Here's how the part is built. I have some questions about the finished solid (model axes, mm). A direction names the side the tool comes from. Coordinates: 2 decimals unless noted, no trailing zeros. Write each loop counter-clockwise with the first axis right and the second up, starting at its lowest first coordinate (ties: lowest second). Pieces come first, ordered by that corner, then holes. Notation, with made-up numbers: (76.25, 9) -> (129.25, 9) arc R16 ccw to (129.25, 29) -> close; hole circle Ø6 at (54, 84.25). An arc over 180 degrees is marked (long way). Use a Markdown table: item, result. Add a question column.
Item 1: If I drill on line 1 along Y through (x, z) = (0, 33.5); line 2 along Z through (x, y) = (-28.5, 17); line 3 along Y through (x, z) = (5, 60), over which ranges is the centre line in solid material (lowest first)? Write a range as from..to.
Item 2: If we mould it in two halves opening along X, with no side actions, what happens to faces 3 (the flat face through (-12, -4, 160)), 4 (the conical face through (34.327, -7.623, 0.243)), 5 (the cylindrical face through (-12.19, 0.54, 78.88))? For each: pulls with the +X half, pulls with the -X half, needs draft (parallel to the pull), parting line crosses it, or undercut.
Item 3: Will these pins go through, and if not, where does the flat tip stop? pin 1 Ø6 at (y, z) = (-1.5, 137) entering from -X; pin 2 Ø2 at (x, y) = (-31.5, -21) entering from +Z; pin 3 Ø12 at (x, z) = (15, 121.5) entering from +Y.
Item 4: On a 3-axis mill with a long thin cutter (end or side, diameter ignored), from which of +Z, -Z, +X, -X, +Y, -Y can I reach the whole of each face in a straight line? I mean faces 1 (the cylindrical face through (-17.183, 0.756, 81.415)), 2 (the flat face through (15, 0, 0)). Say none if no direction works.
Item 5: Imagine slicing it at A-A, the plane x = 0. Write out the boundary of the cut face in (y, z).
Item 6: Imagine slicing it at C-C, the plane z = 28. Write out the boundary of the cut face in (x, y).
```python
from build123d import *

# Parameters (mm, degrees)
F3_DEPTH = 5
F1_R     = 17.2
F4_DEPTH = 160
F0_R     = 12.2
F5_DEPTH = 160


# Not quite as in the source:
# - a fillet or chamfer that OpenCascade refuses, or shapes differently, is made with other operations: its cross-section is extruded or revolved along the edge and cut away or added


with BuildPart() as f3:
    # F2 (on Top) → F3 (new body)
    with BuildSketch(Plane.XY):
        with BuildLine():
            ThreePointArc((40, 0), (28.2842712475, 28.2842712475), (0, 40))
            ThreePointArc((0, 40), (-28.2842712475, 28.2842712475), (-40, 0))
            ThreePointArc((-40, 0), (-28.2842712475, -28.2842712475), (0, -40))
            ThreePointArc((0, -40), (28.2842712475, -28.2842712475), (40, 0))
        make_face()
    extrude(amount=F3_DEPTH)

    # F1 (on Top) → F4 (join)
    with BuildSketch(Plane.XY):
        Circle(F1_R)
    extrude(amount=F4_DEPTH)

    # F0 (on Top) → F5 (cut)
    with BuildSketch(Plane.XY):
        Circle(F0_R)
    extrude(amount=F5_DEPTH, mode=Mode.SUBTRACT)

    # F6: chamfer of 5.08 on 1 edges, made by hand

    # F6_s1 → F6_t2 (revolve, cut)
    with BuildSketch(Plane.YZ):
        Polygon((40, 5.08), (34.92, 0), (40, 0), align=None)
    revolve(axis=Axis((0, 0, 0), (0, 0, 1)), mode=Mode.SUBTRACT)


solid = f3.part
```
Ans:
| question | item | result |
|---|---|---|
| 1 | line 1 | y = -17.2..-12.2, 12.2..17.2 |
| 1 | line 2 | z = 0..5 |
| 1 | line 3 | y = -16.46..-11.13, 11.13..16.46 |
| 2 | face 3 | needs draft |
| 2 | face 4 | parting line crosses it |
| 2 | face 5 | undercut |
| 3 | pin 1 | stops at x = -17.2 |
| 3 | pin 2 | stops at z = 5 |
| 3 | pin 3 | stops at y = 14.66 |
| 4 | face 1 | +Z |
| 4 | face 2 | -Z, +X, -X, +Y, -Y |
| 5 | outline | (-39.92, 5) -> (-34.92, 0) -> (-12.2, 0) -> (-12.2, 160) -> (-17.2, 160) -> (-17.2, 5) -> close; (12.2, 0) -> (34.92, 0) -> (39.92, 5) -> (17.2, 5) -> (17.2, 160) -> (12.2, 160) -> close |
| 6 | outline | circle Ø34.4 at (0, 0); hole circle Ø24.4 at (0, 0) |
